```python
from build123d import *
from build123d.topology import SkipClean

# Parameters (mm, degrees)
BOSS_EXTRUDE1_OUTLINE_R = 4.5
BOSS_EXTRUDE1_DEPTH     = 4
BOSS_EXTRUDE2_START     = -2
BOSS_EXTRUDE2_DEPTH     = 1.2
BOSS_EXTRUDE3_DEPTH     = 2
BOSS_EXTRUDE4_DEPTH     = 2
BOSS_EXTRUDE5_DEPTH     = 2
CUT_EXTRUDE3_DEPTH      = 1.2
SKETCH12_R              = 4
CUT_EXTRUDE4_DEPTH      = 4
SKETCH8_R               = 1.5
CUT_EXTRUDE1_DEPTH      = 56.707591784
CUT_EXTRUDE2_START      = -15
SKETCH9_R               = 4
CUT_EXTRUDE2_DEPTH      = 15


# Read off the part's stored shape, not the designer's step: Boss-Extrude1
with BuildPart() as part:
    # Boss-Extrude1 outline → Boss-Extrude1 (new body)
    with BuildSketch(Plane(origin=(0, 0, 0), x_dir=(-1, 0, 0), z_dir=(0, 0, -1))):
        with BuildLine():
            Line((-7.4, 23.45), (-7.4, 14.446692543))
            ThreePointArc((-7.4, 14.446692543), (-8.012107067, 10.506844717), (-9.790721745, 6.938426891))
            ThreePointArc((-9.790721745, 6.938426891), (-12, 0), (-9.790721745, -6.938426891))
            ThreePointArc((-9.790721745, -6.938426891), (-8.012107067, -10.506844717), (-7.4, -14.446692543))
            Line((-7.4, -14.446692543), (-7.4, -23.45))
            Line((-7.4, -23.45), (7.4, -23.45))
            Line((7.4, -23.45), (7.4, -14.446692543))
            ThreePointArc((7.4, -14.446692543), (8.012107067, -10.506844717), (9.790721745, -6.938426891))
            ThreePointArc((9.790721745, -6.938426891), (12, 0), (9.790721745, 6.938426891))
            ThreePointArc((9.790721745, 6.938426891), (8.012107067, 10.506844717), (7.4, 14.446692543))
            Line((7.4, 14.446692543), (7.4, 23.45))
            Line((7.4, 23.45), (-7.4, 23.45))
        make_face()
        with BuildLine():
            add(Edge.make_bspline(
                [(-5.08661691, -7.066518716), (-5.158505421, -7.088491281), (-5.232048751, -7.104749218), (-5.306303966, -7.11531731)],
                knots=[0, 0, 0, 0, 0.301273824, 0.301273824, 0.301273824, 0.301273824], degree=3))
            ThreePointArc((-5.306303966, -7.11531731), (-6.708944151, -4.587692504), (-4.204222203, -6.030833041))
            add(Edge.make_bspline(
                [(-4.204222203, -6.030833041), (-4.215901752, -6.103480441), (-4.232873947, -6.175405229), (-4.255236782, -6.246594027)],
                knots=[0.717333192, 0.717333192, 0.717333192, 0.717333192, 1, 1, 1, 1], degree=3))
            add(Edge.make_bspline(
                [(-4.255236782, -6.246594027), (-4.333126561, -6.431712412), (-4.447649884, -6.599923699), (-4.729572884, -6.878207782), (-4.900435719, -6.991204718), (-5.08661691, -7.066518716)],
                knots=[0, 0, 0, 0, 0.5, 0.5, 1, 1, 1, 1], degree=3))
        make_face(mode=Mode.SUBTRACT)
        with BuildLine():
            add(Edge.make_bspline(
                [(7.28775176, -8.127178888), (7.215863249, -8.149151453), (7.14231992, -8.16540939), (7.068064705, -8.175977482)],
                knots=[0, 0, 0, 0, 0.301273824, 0.301273824, 0.301273824, 0.301273824], degree=3))
            ThreePointArc((7.068064705, -8.175977482), (5.665424519, -5.648352676), (8.170146468, -7.091493213))
            add(Edge.make_bspline(
                [(8.170146468, -7.091493213), (8.158466918, -7.164140613), (8.141494724, -7.236065401), (8.119131889, -7.307254199)],
                knots=[0.717333192, 0.717333192, 0.717333192, 0.717333192, 1, 1, 1, 1], degree=3))
            add(Edge.make_bspline(
                [(8.119131889, -7.307254199), (8.04124211, -7.492372584), (7.926718787, -7.66058387), (7.644795787, -7.938867954), (7.473932951, -8.05186489), (7.28775176, -8.127178888)],
                knots=[0, 0, 0, 0, 0.5, 0.5, 1, 1, 1, 1], degree=3))
        make_face(mode=Mode.SUBTRACT)
        with BuildLine():
            add(Edge.make_bspline(
                [(-6.147277082, 5.307849955), (-6.219165593, 5.28587739), (-6.292708922, 5.269619453), (-6.366964138, 5.259051361)],
                knots=[0, 0, 0, 0, 0.301273824, 0.301273824, 0.301273824, 0.301273824], degree=3))
            ThreePointArc((-6.366964138, 5.259051361), (-7.769604322, 7.786676168), (-5.264882374, 6.34353563))
            add(Edge.make_bspline(
                [(-5.264882374, 6.34353563), (-5.276561924, 6.27088823), (-5.293534119, 6.198963441), (-5.315896954, 6.127774644)],
                knots=[0.717333192, 0.717333192, 0.717333192, 0.717333192, 1, 1, 1, 1], degree=3))
            add(Edge.make_bspline(
                [(-5.315896954, 6.127774644), (-5.393786733, 5.942656259), (-5.508310056, 5.774444972), (-5.790233055, 5.496160889), (-5.961095891, 5.383163953), (-6.147277082, 5.307849955)],
                knots=[0, 0, 0, 0, 0.5, 0.5, 1, 1, 1, 1], degree=3))
        make_face(mode=Mode.SUBTRACT)
        Circle(BOSS_EXTRUDE1_OUTLINE_R, mode=Mode.SUBTRACT)
        with BuildLine():
            add(Edge.make_bspline(
                [(6.227091589, 4.247189783), (6.155203078, 4.225217218), (6.081659748, 4.208959281), (6.007404533, 4.198391189)],
                knots=[0, 0, 0, 0, 0.301273824, 0.301273824, 0.301273824, 0.301273824], degree=3))
            ThreePointArc((6.007404533, 4.198391189), (4.604764348, 6.726015995), (7.109486296, 5.282875458))
            add(Edge.make_bspline(
                [(7.109486296, 5.282875458), (7.097806747, 5.210228058), (7.080834552, 5.13830327), (7.058471717, 5.067114472)],
                knots=[0.717333192, 0.717333192, 0.717333192, 0.717333192, 1, 1, 1, 1], degree=3))
            add(Edge.make_bspline(
                [(7.058471717, 5.067114472), (6.980581938, 4.881996087), (6.866058615, 4.7137848), (6.584135615, 4.435500717), (6.41327278, 4.322503781), (6.227091589, 4.247189783)],
                knots=[0, 0, 0, 0, 0.5, 0.5, 1, 1, 1, 1], degree=3))
        make_face(mode=Mode.SUBTRACT)
    extrude(amount=BOSS_EXTRUDE1_DEPTH)

    # Sketch4 → Boss-Extrude2 (add)
    with BuildSketch(Plane(origin=(0, -23.45, 0), x_dir=(-1, 0, 0), z_dir=(0, -1, 0)).offset(BOSS_EXTRUDE2_START)):
        with BuildLine():
            Line((-7.4, 4), (-7.4, 22.110096084))
            ThreePointArc((-7.4, 22.110096084), (0, 29.510096084), (7.4, 22.110096084))
            Line((7.4, 22.110096084), (7.4, 4))
            Line((7.4, 4), (-7.4, 4))
        make_face()
    boss_extrude2 = extrude(amount=-BOSS_EXTRUDE2_DEPTH)

    # Mirror1: Boss-Extrude2 across plane
    add(boss_extrude2.mirror(Plane.ZX))

    # Sketch6 → Boss-Extrude3 (add)
    with BuildSketch(Plane.XZ.offset(21.45)):
        with BuildLine():
            ThreePointArc((-7.4, -22.110096084), (0, -29.510096084), (7.4, -22.110096084))
            Line((7.4, -22.110096084), (7.4, -4))
            Line((7.4, -4), (-7.4, -4))
            Line((-7.4, -4), (-7.4, -22.110096084))
        make_face()
        with BuildLine():
            Line((-3.920792079, -21.318016876), (-2.5, -7.110096084))
            ThreePointArc((-2.5, -7.110096084), (0, -4.610096084), (2.5, -7.110096084))
            Line((2.5, -7.110096084), (3.920792079, -21.318016876))
            ThreePointArc((3.920792079, -21.318016876), (3.980148761, -21.712081207), (4, -22.110096084))
            ThreePointArc((4, -22.110096084), (0, -26.110096084), (-4, -22.110096084))
            ThreePointArc((-4, -22.110096084), (-3.980148761, -21.712081207), (-3.920792079, -21.318016876))
        make_face(mode=Mode.SUBTRACT)
    extrude(amount=BOSS_EXTRUDE3_DEPTH)

    # Sketch7 → Boss-Extrude4 (add)
    with BuildSketch(Plane(origin=(0, 21.45, 0), x_dir=(1, 0, 0), z_dir=(0, 1, 0))):
        with BuildLine():
            Line((-7.4, 22.110096084), (-7.4, 4))
            Line((-7.4, 4), (7.4, 4))
            Line((7.4, 4), (7.4, 22.110096084))
            ThreePointArc((7.4, 22.110096084), (0, 29.510096084), (-7.4, 22.110096084))
        make_face()
    extrude(amount=BOSS_EXTRUDE4_DEPTH)

    # Sketch10 → Boss-Extrude5 (add)
    with BuildSketch(Plane.XZ.offset(-20.25)):
        with BuildLine():
            Line((7.4, -4), (-7.4, -4))
            Line((-7.4, -4), (-7.4, -22.110096084))
            ThreePointArc((-7.4, -22.110096084), (0, -29.510096084), (7.4, -22.110096084))
            Line((7.4, -22.110096084), (7.4, -4))
        make_face()
    extrude(amount=BOSS_EXTRUDE5_DEPTH)

    # Sketch11 → Cut-Extrude3 (cut)
    with BuildSketch(Plane(origin=(0, 23.45, 0), x_dir=(1, 0, 0), z_dir=(0, 1, 0))):
        with BuildLine():
            Line((-7.4, 0), (7.4, 0))
            Line((7.4, 0), (7.4, 22.110096084))
            ThreePointArc((7.4, 22.110096084), (0, 29.510096084), (-7.4, 22.110096084))
            Line((-7.4, 22.110096084), (-7.4, 0))
        make_face()
    extrude(amount=-CUT_EXTRUDE3_DEPTH, mode=Mode.SUBTRACT)

    # Sketch12 → Cut-Extrude4 (cut)
    with BuildSketch(Plane(origin=(0, 22.25, 0), x_dir=(1, 0, 0), z_dir=(0, 1, 0))):
        with Locations(Location((0, 22.110096084, 0), (0, 0, 270))):
            Circle(SKETCH12_R)
    extrude(amount=-CUT_EXTRUDE4_DEPTH, mode=Mode.SUBTRACT)

    # Sketch8 → Cut-Extrude1 (cut, through all)
    with BuildSketch(Plane.XZ.offset(23.45)):
        with Locations(Location((0, -22.110096084, 0), (0, 0, 270))):
            Circle(SKETCH8_R)
    extrude(amount=-CUT_EXTRUDE1_DEPTH, mode=Mode.SUBTRACT)

    # Sketch9 → Cut-Extrude2 (cut)
    with SkipClean():  # the faces are left unmerged after this step: merging them gives an invalid solid
        with BuildSketch(Plane.XZ.offset(23.45).offset(CUT_EXTRUDE2_START)):
            with Locations(Location((0, -22.110096084, 0), (0, 0, 11.421186275))):
                Circle(SKETCH9_R)
        extrude(amount=CUT_EXTRUDE2_DEPTH, mode=Mode.SUBTRACT)


solid = part.part
```
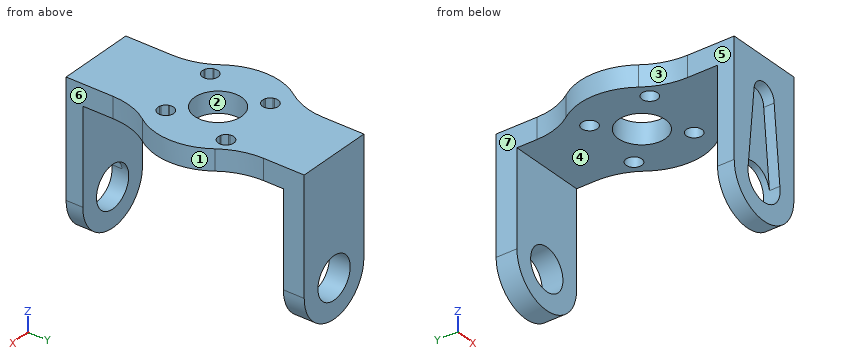
The model under review builds one solid part; all positions refer to its coordinate system, in mm. Face numbers are marked on the shaded views. A direction names the side the tool comes from. Round coordinates to 2 decimals unless told otherwise and drop trailing zeros. Loops run counter-clockwise (first coordinate to the right, second up) from the corner with the lowest first, then second, coordinate; pieces in that order, holes last. Notation, with made-up numbers: (37.5, -10) - (87.5, -10) arc R33 ccw to (87.5, 20) - close; hole circle Ø9 at (71, -18). An arc over 180 degrees is marked (long way). Write each question's results on one line, items separated by ' | '. Start each with the question number.
Q1. Take a section at B-B on x = 0. Give the boundary of the cut face in (y, z), plus the area to 3 significant figures.
Q2. Insertion check: P1, Ø8, axis at x = -9.5, y = 12.5, coming from the -Z side; P2, Ø2, axis at x = -9, z = -5.5, coming from the -Y side; P3, Ø12, axis at x = 1, z = -21.5, coming from the -Y side; P4, Ø8.5, axis at y = 19, z = -8, coming from the -X side. Each pin has a flat end and moves straight along its axis. Give the tip position at first contact, or say it passes through.
Q3. Take a section at C-C on z = -5.25. Give the boundary of the cut face in (x, y).
Q4. Take a section at A-A on y = 0. Give the boundary of the cut face in (x, z).
Q5. Tool access review of the marked faces 4, 5, 6 and 7: name each direction out of +Z, -Z, +X, -X, +Y, -Y from which nothing blocks a thin tool from reaching the whole face with its end or side.
Q6. Wall thickness on line 1 along Y through (x, z) = (-5.75, -6.75); line 2 along Z through (x, y) = (0, -22.05); line 3 along X through (y, z) = (20, -17.25): over which ranges is each line inside the solid? List them lowest first. Write a range as [from, to].
Q7. Draft analysis for pull direction X (two halves, no side actions). For the marked faces 1, 2 and 3, state which applies: pulls with the +X half, pulls with the -X half, needs draft (parallel to the pull), parting line crosses it, or undercut.
Q8. Take a section at D-D on z = -19.75. Give the boundary of the cut face in (x, y), plus the area to 3 significant figures.
Data:
1) outline: (-23.45, -29.51) - (-20.25, -29.51) - (-20.25, -26.11) - (-23.45, -26.11) - close; (-23.45, -4.61) - (-21.45, -4.61) - (-21.45, -18.11) - (-20.25, -18.11) - (-20.25, -4) - (-4.5, -4) - (-4.5, 0) - (-23.45, 0) - close; (4.5, -4) - (18.25, -4) - (18.25, -18.11) - (22.25, -18.11) - (22.25, 0) - (4.5, 0) - close; (18.25, -29.51) - (22.25, -29.51) - (22.25, -26.11) - (18.25, -26.11) - close | area: 246 mm²
2) P1: stops at z = -4 | P2: passes through | P3: stops at y = -23.45 | P4: stops at x = -7.4
3) outline: (-7.4, -23.45) - (-1.67, -23.45) - (-1.67, -21.45) - (1.67, -21.45) - (1.67, -23.45) - (7.4, -23.45) - (7.4, -20.25) - (-7.4, -20.25) - close; (-7.4, 18.25) - (7.4, 18.25) - (7.4, 22.25) - (-7.4, 22.25) - close
4) outline: (-12, -4) - (-4.5, -4) - (-4.5, 0) - (-12, 0) - close; (4.5, -4) - (12, -4) - (12, 0) - (4.5, 0) - close
5) face 4: -Z, +X, -X | face 5: +Z, -Z, -X, -Y | face 6: +Z, -Z, +X, -Y | face 7: +Z, -Z, -X, +Y
6) line 1: y = [-23.45, -20.25], [18.25, 22.25] | line 2: z = [-29.51, -26.11], [-4.61, 0] | line 3: x = [-7.4, 7.4]
7) face 1: pulls with the +X half | face 2: undercut | face 3: pulls with the -X half
8) outline: (-7.4, -23.45) - (-3.76, -23.45) - (-3.76, -21.45) - (-3.23, -21.45) - (-3.23, -20.25) - (-7.4, -20.25) - close; (-7.4, 18.25) - (-3.23, 18.25) - (-3.23, 22.25) - (-7.4, 22.25) - close; (3.23, -21.45) - (3.76, -21.45) - (3.76, -23.45) - (7.4, -23.45) - (7.4, -20.25) - (3.23, -20.25) - close; (3.23, 18.25) - (7.4, 18.25) - (7.4, 22.25) - (3.23, 22.25) - close | area: 57.9 mm²
